```python
from build123d import *

# Parameters (mm, degrees)
SKETCH1_W       = 6
SKETCH1_H       = 12
EXTRUDE1_DEPTH  = 6
SKETCH3_W       = 4
SKETCH3_H       = 8.6
EXTRUDE2_DEPTH  = 1
SKETCH2_R       = 1.25
EXTRUDE3_DEPTH  = 5.5
EXTRUDE4_DEPTH  = 4
SKETCH6_R       = 8.5
EXTRUDE5_DEPTH  = 4
FILLET1_R       = 4
EXTRUDE9_START  = -4
EXTRUDE9_DEPTH  = 4
EXTRUDE10_DEPTH = 2
SKETCH14_R      = 1.25
EXTRUDE11_DEPTH = 4


with BuildPart() as part:
    # Sketch1 → Extrude1 (new body)
    with BuildSketch(Plane.XY):
        with Locations((-1, 0)):
            Rectangle(SKETCH1_W, SKETCH1_H)
    extrude(amount=EXTRUDE1_DEPTH)

    # Sketch3 → Extrude2 (add)
    with BuildSketch(Plane.XY.offset(6)):
        Rectangle(SKETCH3_W, SKETCH3_H)
    extrude(amount=EXTRUDE2_DEPTH)

    # Sketch2 → Extrude3 (cut)
    with BuildSketch(Plane(origin=(0, 0, 0), x_dir=(-1, 0, 0), z_dir=(0, 0, -1))):
        with Locations((1, 3)):
            Circle(SKETCH2_R)
        with Locations((1, -3)):
            Circle(SKETCH2_R)
    extrude(amount=-EXTRUDE3_DEPTH, mode=Mode.SUBTRACT)

    # Sketch4 → Extrude4 (add)
    with BuildSketch(Plane(origin=(2, 0, 0), x_dir=(0, 0, -1), z_dir=(1, 0, 0))):
        with BuildLine():
            Line((-7, 6), (-6, 6))
            Line((-6, 6), (-6, -6))
            Line((-6, -6), (-7, -6))
            ThreePointArc((-7, -6), (-25, 0), (-7, 6))
        make_face()
    extrude(amount=-EXTRUDE4_DEPTH)

    # Sketch6 → Extrude5 (cut)
    with BuildSketch(Plane.ZY.offset(2)):
        with Locations(Location((15, 0, 0), (0, 0, 270))):
            Circle(SKETCH6_R)
    extrude(amount=-EXTRUDE5_DEPTH, mode=Mode.SUBTRACT)

    # Fillet1
    # the kernel refuses this fillet: 4 mm, written as the material it adds along each edge
    with BuildSketch(Plane(origin=(2, 6, 7), x_dir=(0, 0, -1), z_dir=(-1, 0, 0))) as fillet1_piece_1_section:
        with BuildLine():
            CenterArc((1.797958971, -4), FILLET1_R, 90, 44.415308597)
            ThreePointArc((-1.001457878, -1.142857143), (-0.478989625, -0.590478203), (0, 0))
            Line((0, 0), (1.797958971, 0))
        make_face()
    fillet1_piece_1 = extrude(amount=4, mode=Mode.PRIVATE)
    fillet1_piece_1 = split(fillet1_piece_1, bisect_by=Plane(origin=(0, 5.976030652, 6), z_dir=(0, 0, -1)), keep=Keep.TOP, mode=Mode.PRIVATE)
    add(fillet1_piece_1)
    with BuildSketch(Plane(origin=(2, 6, 7), x_dir=(0, 0, -1), z_dir=(-1, 0, 0))) as fillet1_piece_2_section:
        with BuildLine():
            CenterArc((1.797958971, -4), FILLET1_R, 90, 44.415308597)
            ThreePointArc((-1.001457878, -1.142857143), (-0.478989625, -0.590478203), (0, 0))
            Line((0, 0), (1.797958971, 0))
        make_face()
    fillet1_piece_2 = extrude(amount=4, mode=Mode.PRIVATE)
    fillet1_piece_2 = split(fillet1_piece_2, bisect_by=Plane(origin=(0, 6.277319808, 6), z_dir=(0, 0, 1)), keep=Keep.TOP, mode=Mode.PRIVATE)
    add(fillet1_piece_2)
    with BuildSketch(Plane(origin=(2, 6, 7), x_dir=(0, 0, -1), z_dir=(-1, 0, 0))) as fillet1_piece_3_section:
        with BuildLine():
            CenterArc((1.797958971, -4), FILLET1_R, 90, 44.415308597)
            ThreePointArc((-1.001457878, -1.142857143), (-0.478989625, -0.590478203), (0, 0))
            Line((0, 0), (1.797958971, 0))
        make_face()
    fillet1_piece_3 = extrude(amount=8.494897428, mode=Mode.PRIVATE)
    fillet1_piece_3 = split(fillet1_piece_3, bisect_by=Plane(origin=(-4, 5.976030652, 5.651028554), z_dir=(1, 0, 0)), keep=Keep.TOP, mode=Mode.PRIVATE)
    fillet1_piece_3 = split(fillet1_piece_3, bisect_by=Plane(origin=(-3, 5.976030652, 6), z_dir=(0, 0, -1)), keep=Keep.TOP, mode=Mode.PRIVATE)
    fillet1_piece_3 = split(fillet1_piece_3, bisect_by=Plane(origin=(-2, 5.976030652, 5.651028554), z_dir=(-1, 0, 0)), keep=Keep.TOP, mode=Mode.PRIVATE)
    add(fillet1_piece_3)
    with BuildSketch(Plane(origin=(2, -6, 7), x_dir=(0, -0.7521010374968901, 0.6590478202650409), z_dir=(-1, 0, 0))) as fillet1_piece_4_section:
        with BuildLine():
            CenterArc((1.823463209, -3.988438089), FILLET1_R, 94.357396878, 44.415308597)
            Line((-1.184940941, -1.352246808), (0, 0))
            ThreePointArc((0, 0), (0.759776337, -0.028904778), (1.519552674, 0))
        make_face()
    fillet1_piece_4 = extrude(amount=4, mode=Mode.PRIVATE)
    fillet1_piece_4 = split(fillet1_piece_4, bisect_by=Plane(origin=(0, -6.277319808, 6), z_dir=(0, 0, 1)), keep=Keep.TOP, mode=Mode.PRIVATE)
    add(fillet1_piece_4)
    with BuildSketch(Plane(origin=(2, -6, 7), x_dir=(0, -0.7521010374968901, 0.6590478202650409), z_dir=(-1, 0, 0))) as fillet1_piece_5_section:
        with BuildLine():
            CenterArc((1.823463209, -3.988438089), FILLET1_R, 94.357396878, 44.415308597)
            Line((-1.184940941, -1.352246808), (0, 0))
            ThreePointArc((0, 0), (0.759776337, -0.028904778), (1.519552674, 0))
        make_face()
    fillet1_piece_5 = extrude(amount=4, mode=Mode.PRIVATE)
    fillet1_piece_5 = split(fillet1_piece_5, bisect_by=Plane(origin=(0, -5.976030652, 6), z_dir=(0, 0, -1)), keep=Keep.TOP, mode=Mode.PRIVATE)
    add(fillet1_piece_5)
    with BuildSketch(Plane(origin=(2, -6, 7), x_dir=(0, -0.7521010374968901, 0.6590478202650409), z_dir=(-1, 0, 0))) as fillet1_piece_6_section:
        with BuildLine():
            CenterArc((1.823463209, -3.988438089), FILLET1_R, 94.357396878, 44.415308597)
            Line((-1.184940941, -1.352246808), (0, 0))
            ThreePointArc((0, 0), (0.759776337, -0.028904778), (1.519552674, 0))
        make_face()
    fillet1_piece_6 = extrude(amount=8.494897428, mode=Mode.PRIVATE)
    fillet1_piece_6 = split(fillet1_piece_6, bisect_by=Plane(origin=(-4, -5.976030652, 5.651028554), z_dir=(1, 0, 0)), keep=Keep.TOP, mode=Mode.PRIVATE)
    fillet1_piece_6 = split(fillet1_piece_6, bisect_by=Plane(origin=(-3, -5.976030652, 6), z_dir=(0, 0, -1)), keep=Keep.TOP, mode=Mode.PRIVATE)
    fillet1_piece_6 = split(fillet1_piece_6, bisect_by=Plane(origin=(-2, -5.976030652, 5.651028554), z_dir=(-1, 0, 0)), keep=Keep.TOP, mode=Mode.PRIVATE)
    add(fillet1_piece_6)

    # Sketch12 → Extrude9 (add)
    with BuildSketch(Plane.ZY.offset(2).offset(EXTRUDE9_START)):
        with BuildLine():
            Line((18.92820323, -9.196152423), (23.942490318, -12.091152423))
            Line((23.942490318, -12.091152423), (29.942490318, -1.698847577))
            Line((29.942490318, -1.698847577), (24.92820323, 1.196152423))
            ThreePointArc((24.92820323, 1.196152423), (23.660254038, -5), (18.92820323, -9.196152423))
        make_face()
    extrude(amount=EXTRUDE9_DEPTH)

    # Sketch13 → Extrude10 (add)
    with BuildSketch(Plane.ZY.offset(2)):
        Polygon((29.942490318, -1.698847577), (26.045376001, 0.551152423), (20.045376001, -9.841152423), (23.942490318, -12.091152423), align=None)
    extrude(amount=EXTRUDE10_DEPTH)

    # Sketch14 → Extrude11 (cut)
    with BuildSketch(Plane(origin=(0, -13.390190528, 23.192490318), x_dir=(1, 0, 0), z_dir=(0, -0.5000000000000007, 0.8660254037844383))):
        with Locations(Location((-1, 4.5, 0), (0, 0, 270))):
            Circle(SKETCH14_R)
        with Locations(Location((-1, 10.5, 0), (0, 0, 270))):
            Circle(SKETCH14_R)
    extrude(amount=-EXTRUDE11_DEPTH, mode=Mode.SUBTRACT)


solid = part.part
```
Input: part model. Units: mm. Frame: model coordinates. A direction names the side the tool comes from. Give positions to 0.01 mm unless a question says otherwise; leave off trailing zeros. Order: outer loops, then holes, each group sorted by start corner. A loop starts at its lowest first (then second) coordinate and runs counter-clockwise, first axis right, second up. Notation, with made-up numbers: M -18,32 L 9,32 A21 cw 9,41 Z; hole C -5,-37.75 d3. An arc over 180 degrees is marked long. One line per question, with ' | ' between items.
1) Section C-C on z = 11.5. Output: boundary loops of the cut face in (x, y), and give its area (3 significant figures).
Filled in:
outline: M -2,-9.37 L 2,-9.37 L 2,-7.75 L -2,-7.75 Z; M -2,7.75 L 2,7.75 L 2,9.37 L -2,9.37 Z | area: 13.0 mm2
2) Access query for faces 1 (the face through (-1, 3, 5.5)), 2 (the face through (-2, -1, 24)), 3 (the face through (-1, 6, 3)). Directions: +Z, -Z, +X, -X, +Y, -Y. A direction counts if a zero-diameter tool reaches every point of the face in a straight line with its end or side. Return the directions, or none.
Filled in:
face 1: -Z | face 2: -X, +Y | face 3: -Z, +X, -X, +Y
3) Draft query along Y for faces 4 (the face through (-0.96, -6.97, 26.9)), 5 (the face through (-1, -3, 5.5)), 6 (the face through (-4, -6, 25)), 7 (the face through (-1.76, -7.65, 24.23)). Return one class per face: pulls with the +Y half, pulls with the -Y half, needs draft (parallel to the pull), parting line crosses it, or undercut.
Filled in:
face 4: pulls with the -Y half | face 5: undercut | face 6: needs draft | face 7: undercut
4) Section D-D on x = -1. Output: boundary loops of the cut face in (y, z), and give its area (3 significant figures).
Filled in:
outline: M -12.09,23.94 L -9.2,18.93 A10 ccw -7.14,8 A4 cw -6,5.2 L -6,0 L -4.25,0 L -4.25,5.5 L -1.75,5.5 L -1.75,0 L 1.75,0 L 1.75,5.5 L 4.25,5.5 L 4.25,0 L 6,0 L 6,5.2 A4 cw 7.14,8 A10 ccw 1.2,24.93 L -1.7,29.94 L -3.21,29.07 L -1.21,25.6 L -3.38,24.35 L -5.38,27.82 L -8.41,26.07 L -6.41,22.6 L -8.58,21.35 L -10.58,24.82 Z; hole C 0,15 d17 | area: 161 mm2
5) Contact query for flat-ended pins moving along their axis: P1, Ø3, axis at x = -1, y = 3, coming from the +Z side; P2, Ø3, axis at x = -1, y = -3, coming from the +Z side; P3, Ø3, axis at x = -0.5, z = 3.5, coming from the -Y side. Output: stop coordinate, or through.
Filled in:
P1: stops at z = 24.89 | P2: stops at z = 29.94 | P3: stops at y = -6
6) Ray query, L1, parallel to Y at x = -1, z = 4.1; L2, parallel to Y at x = 1.8, z = 4.75; L3, parallel to Z at x = -1.8, y = 7.75. Return the intervals inside material, ascending.
Filled in:
L1: y = -6 to -4.25, -1.75 to 1.75, 4.25 to 6 | L2: y = -6 to 6 | L3: z = 8.68 to 11.51, 18.49 to 21.32
7) Section A-A on x = -2.85. Output: boundary loops of the cut face in (y, z), and give its area (3 significant figures).
Filled in:
outline: M -12.09,23.94 L -9.84,20.05 L 0.55,26.05 L -1.7,29.94 Z; M -6.08,6 A4 cw -6,5.2 L -6,0 L 6,0 L 6,5.2 A4 cw 6.08,6 Z | area: 126 mm2
8) Section B-B on y = 7.75. Output: boundary loops of the cut face in (x, z).
Filled in:
outline: M -2,8.68 L 2,8.68 L 2,11.51 L -2,11.51 Z; M -2,18.49 L 2,18.49 L 2,21.32 L -2,21.32 Z
